Build history of the part. All positions in model axes, mm. A direction names the side the tool comes from. Coordinates: 2 decimals unless noted, no trailing zeros. Order: outer loops, then holes, each group sorted by start corner. A loop starts at its lowest first (then second) coordinate and runs counter-clockwise, first axis right, second up. Notation, with made-up numbers: (76, -9) - (84, -9) arc R31 ccw to (84, 24) - close; hole circle Ø8 at (20, -16.5). An arc over 180 degrees is marked (long way). One line per item, written item: value.
from build123d import *

# Parameters (mm, degrees)
F0_R          = 5
F1_DEPTH      = 18.75
F1_DEPTH_BACK = 18.75
F4_DEPTH      = 7
F4_DEPTH_BACK = 7
F6_R          = 7.5
F7_DEPTH      = 150
F8_R          = 2.49999


# Not quite as in the source:
# - a fillet or chamfer is up to 0.001 mm smaller than in the source, because OpenCascade refuses the exact size
# - a feature names something its author has since deleted; it is built from what else it names


with BuildPart() as f1:
    # F0 (on Front) → F1 (new body, two sides)
    with BuildSketch(Plane.XZ) as f1_sk:
        with BuildLine():
            Line((10, 0), (10, 20))
            ThreePointArc((10, 20), (0, 30), (-10, 20))
            Line((-10, 20), (-10, 0))
            Line((-10, 0), (10, 0))
        make_face()
        with Locations((0, 20)):
            Circle(F0_R, mode=Mode.SUBTRACT)
    extrude(amount=F1_DEPTH)
    extrude(f1_sk.sketch, amount=-F1_DEPTH_BACK)

    # F3 (on offset) → F4 (cut, two sides)
    with BuildSketch(Plane.XZ) as f4_sk:
        Polygon((-12, 5), (0, 5), (12, 5), (12, 35), (-12, 35), align=None)
    extrude(amount=-F4_DEPTH, mode=Mode.SUBTRACT)
    extrude(f4_sk.sketch, amount=F4_DEPTH_BACK, mode=Mode.SUBTRACT)

    # F6 (on offset) → F7 (join)
    with BuildSketch(Plane(origin=(0, 0, 0), x_dir=(1, 0, 0), z_dir=(0, 0, -1))):
        Circle(F6_R)
    extrude(amount=F7_DEPTH)

    # F8 (radius 2.5 in the source; OpenCascade refuses exactly that, so slightly less here)
    f8_edges = [f1.edges().sort_by_distance(p)[0] for p in [
        (10, -7, 12.5),
        (10, 7, 12.5),
        (10, 18.75, 10),
        (10, -18.75, 10),
        (10, 0, 5),
        (-10, 0, 5),
        (10, 0, 0),
        (0, 18.75, 0),
        (0, -18.75, 0),
    ]]
    fillet(f8_edges, radius=F8_R)


solid = f1.part
1. 3-axis set-ups, long thin cutter, end or side, ignore diameter. For faces 1 (the face through (0, 0, 5)), 2 (the face through (0, -13, 30)), 3 (the face through (-7.493, -0.33, -73.95)): which of +Z, -Z, +X, -X, +Y, -Y reach the whole face in a straight line?
Values found:
face 1: +Z, +X, -X
face 2: +Z, +Y, -Y
face 3: -Z
2. Band-saw the part on B-B, the plane z = 12. Give the cut face in (x, y).
Values found:
outline: (-10, -16.25) arc R2.5 ccw to (-7.5, -18.75) - (7.5, -18.75) arc R2.5 ccw to (10, -16.25) - (10, -9.5) arc R2.5 ccw to (7.5, -7) - (-7.5, -7) arc R2.5 ccw to (-10, -9.5) - close; (-10, 9.5) arc R2.5 ccw to (-7.5, 7) - (7.5, 7) arc R2.5 ccw to (10, 9.5) - (10, 16.25) arc R2.5 ccw to (7.5, 18.75) - (-7.5, 18.75) arc R2.5 ccw to (-10, 16.25) - close
3. Band-saw the part on D-D, the plane z = -32.5. Give the cut face in (x, y).
Values found:
outline: circle Ø15 at (0, 0)
4. Flat gauge pins, fed straight in: P1, Ø4, axis at x = -2.5, y = 11.5, coming from the -Z side; P2, Ø4, axis at x = -3, y = -2.5, coming from the +Z side; P3, Ø8, axis at x = 0, z = 20, coming from the -Y side; P4, Ø3, axis at y = 7.5, z = -99.5, coming from the +X side. Where does each tip first touch, or does it go through?
Values found:
P1: stops at z = 0
P2: stops at z = 5
P3: passes through
P4: stops at x = 4.5
5. Band-saw the part on A-A, the plane x = 0. Give the cut face in (y, z), and give its area (3 significant figures).
Values found:
outline: (-18.75, 2.5) arc R2.5 ccw to (-16.25, 0) - (-7.5, 0) - (-7.5, -150) - (7.5, -150) - (7.5, 0) - (16.25, 0) arc R2.5 ccw to (18.75, 2.5) - (18.75, 15) - (7, 15) - (7, 5) - (-7, 5) - (-7, 15) - (-18.75, 15) - close; (-18.75, 25) - (-7, 25) - (-7, 27.5) arc R2.5 ccw to (-9.5, 30) - (-16.25, 30) arc R2.5 ccw to (-18.75, 27.5) - close; (7, 25) - (18.75, 25) - (18.75, 27.5) arc R2.5 ccw to (16.25, 30) - (9.5, 30) arc R2.5 ccw to (7, 27.5) - close
area: 2,780 mm2
6. Two-plate mould, pull along X, no slides. Class faces 4 (the face through (-1.08, 12.79, 15.12)), 5 (the face through (0, -7, 14)), 6 (the face through (-10, 0, 1)): pulls with the +X half, pulls with the -X half, needs draft (parallel to the pull), parting line crosses it, or undercut.
Values found:
face 4: undercut
face 5: needs draft
face 6: pulls with the -X half
7. Probe line 1 along Z through (x, y) = (0, -12.5); line 2 along X through (y, z) = (-16, 20); line 3 along Y through (x, z) = (7.75, 20). List the from-to ranges inside material, lowest first.
Values found:
line 1: z = 0 to 15, 25 to 30
line 2: x = -10 to -5, 5 to 10
line 3: y = -18.74 to -7.01, 7.01 to 18.74
